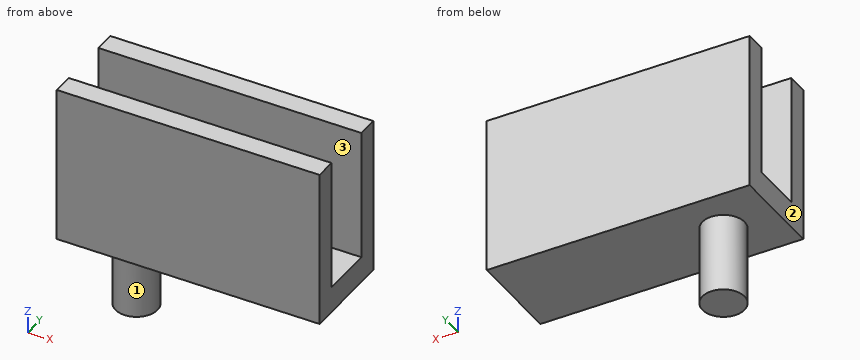
from build123d import *

# Parameters (mm, degrees)
F0_R     = 4
F1_DEPTH = 15
F2_W     = 50
F2_H     = 18
F2_R     = 4
F3_DEPTH = 30
F4_W     = 50
F4_H     = 25
F5_DEPTH = 5


with BuildPart() as f1:
    # F0 (on Top) → F1 (new body)
    with BuildSketch(Plane.XY):
        with Locations((0, 0.135727)):
            Circle(F0_R)
    extrude(amount=F1_DEPTH)

    # F2 (on face) → F3 (join)
    with BuildSketch(Plane.XY.offset(15)):
        with Locations((15, 0)):
            Rectangle(F2_W, F2_H)
        with Locations((0, 0.135727)):
            Circle(F2_R, mode=Mode.SUBTRACT)
        with Locations((0, 0.135727)):
            Circle(F2_R)
    extrude(amount=F3_DEPTH)

    # F4 (on Front) → F5 (cut, symmetric)
    with BuildSketch(Plane.XZ):
        with Locations((15, 32.5)):
            Rectangle(F4_W, F4_H)
    extrude(amount=F5_DEPTH, both=True, mode=Mode.SUBTRACT)


solid = f1.part
Can you work these out from the model? Positions are in its coordinate system, mm. Face numbers are marked on the shaded views. A direction names the side the tool comes from. Coordinates: 2 decimals unless noted, no trailing zeros. Write each loop counter-clockwise with the first axis right and the second up, starting at its lowest first coordinate (ties: lowest second). Pieces come first, ordered by that corner, then holes.
Q1. Which directions (+Z, -Z, +X, -X, +Y, -Y) give clear straight access to the entire face, cutting with the end or side of a thin tool? Please do the marked faces 1, 2 and 3.
Results found:
face 1: -Z
face 2: +Z, -Z, -X, +Y, -Y
face 3: +Z, +X, -X
Q2. Please list where these lines run through material, in increasing order: L1, parallel to Y at x = 12, z = 39; L2, parallel to Z at x = 3, y = 6.5; L3, parallel to Z at x = -3.5, y = -4.25.
Results found:
L1: y = -9 to -5, 5 to 9
L2: z = 15 to 45
L3: z = 15 to 20
Q3. Imagine slicing it at A-A, the plane z = 35.5. List the corners of the cut face in (x, y) for me.
Results found:
outline: (-10, -9) - (40, -9) - (40, -5) - (-10, -5) - close; (-10, 5) - (40, 5) - (40, 9) - (-10, 9) - close
Q4. Imagine slicing it at D-D, the plane x = 0. List the corners of the cut face in (y, z) for me.
Results found:
outline: (-9, 15) - (-3.86, 15) - (-3.86, 0) - (4.14, 0) - (4.14, 15) - (9, 15) - (9, 45) - (5, 45) - (5, 20) - (-5, 20) - (-5, 45) - (-9, 45) - close
Q5. Imagine slicing it at C-C, the plane y = 1. List the corners of the cut face in (x, z) for me.
Results found:
outline: (-10, 15) - (-3.91, 15) - (-3.91, 0) - (3.91, 0) - (3.91, 15) - (40, 15) - (40, 20) - (-10, 20) - close
Q6. Imagine slicing it at B-B, the plane x = 34. List the corners of the cut face in (y, z) for me.
Results found:
outline: (-9, 15) - (9, 15) - (9, 45) - (5, 45) - (5, 20) - (-5, 20) - (-5, 45) - (-9, 45) - close
Q7. For P1, Ø3, axis at x = 17, y = -0.5, coming from the +Z side; P2, Ø1.5, axis at x = 22.5, y = -1, coming from the -Z side, each with a flat end and sliding along its axis, tell me the tip position at first contact or that it passes through.
Results found:
P1: stops at z = 20
P2: stops at z = 15
